```python
from build123d import *

# Parameters (mm, degrees)
SKETCH1_R           = 10
BOSS_EXTRUDE1_DEPTH = 7
SKETCH2_R           = 10
BOSS_EXTRUDE2_DEPTH = 4
SKETCH3_R           = 7
BOSS_EXTRUDE3_DEPTH = 19
SKETCH4_R           = 3
CUT_EXTRUDE1_DEPTH  = 31
CHAMFER1_SIZE       = 0.5
CUT_EXTRUDE2_START  = 10.2
CUT_EXTRUDE2_DEPTH  = 5.8


with BuildPart() as part:
    # Sketch1 → Boss-Extrude1 (new body)
    with BuildSketch(Plane(origin=(0, 0, 0), x_dir=(0, 0, -1), z_dir=(1, 0, 0))):
        Circle(SKETCH1_R)
    extrude(amount=BOSS_EXTRUDE1_DEPTH)

    # Sketch2 → Boss-Extrude2 (add)
    with BuildSketch(Plane(origin=(7, 0, 0), x_dir=(0, 0, -1), z_dir=(1, 0, 0))):
        with Locations((0, 5)):
            Circle(SKETCH2_R)
    extrude(amount=BOSS_EXTRUDE2_DEPTH)

    # Sketch3 → Boss-Extrude3 (add)
    with BuildSketch(Plane(origin=(11, 0, 0), x_dir=(0, 0, -1), z_dir=(1, 0, 0))):
        with Locations((0, 5)):
            Circle(SKETCH3_R)
    extrude(amount=BOSS_EXTRUDE3_DEPTH)

    # Sketch4 → Cut-Extrude1 (cut, through all)
    with BuildSketch(Plane(origin=(30, 0, 0), x_dir=(0, 0, -1), z_dir=(1, 0, 0))):
        with Locations((0, 5)):
            Circle(SKETCH4_R)
    extrude(amount=-CUT_EXTRUDE1_DEPTH, mode=Mode.SUBTRACT)

    # Chamfer1
    chamfer1_edges = [part.edges().sort_by_distance(p)[0] for p in [
        (0, 5, 3),
        (30, 5, 3),
    ]]
    chamfer(chamfer1_edges, length=CHAMFER1_SIZE)

    # Sketch5 → Cut-Extrude2 (cut, through all)
    with BuildSketch(Plane(origin=(0, 0, 0), x_dir=(1, 0, 0), z_dir=(0, 1, 0)).offset(CUT_EXTRUDE2_START)):
        with BuildLine():
            Line((31, 2.5), (18.5, 2.5))
            ThreePointArc((18.5, 2.5), (16, 0), (18.5, -2.5))
            Line((18.5, -2.5), (31, -2.5))
            Line((31, -2.5), (31, 2.5))
        make_face()
    extrude(amount=CUT_EXTRUDE2_DEPTH, mode=Mode.SUBTRACT)


solid = part.part
```
Input: part model. Units: mm. Frame: model coordinates. A direction names the side the tool comes from. Give positions to 0.01 mm unless a question says otherwise; leave off trailing zeros. Loops run counter-clockwise (first coordinate to the right, second up) from the corner with the lowest first, then second, coordinate; pieces in that order, holes last. Notation, with made-up numbers: M -11.75,-38.75 L 10.25,-38.75 A14 cw 10.25,-21.75 Z; hole C 83.25,31.25 d4. An arc over 180 degrees is marked long. Answer as CSV lines item,"result". Start each with the question number.
1. Reachability of faces 4 (the face through (20.37, -1.21, -3.23)), 5 (the face through (7, -6, 0)), 6 (the face through (24, 11, 2.5)), 7 (the face through (7, 10.2, 0.1)) from +Z, -Z, +X, -X, +Y, -Y: full face, straight path, thin tool, end or side. Return the list, or none.
2. Section B-B on x = 20. Return loops of the section in (y, z), plus the area to 3 significant figures.
3. Pull-direction query (Z, two-part tool) for faces 1 (the face through (3.45, -9.76, 2.17)), 2 (the face through (0, 0, 0)), 3 (the face through (15.2, 2.07, 0.65)); classes: released by +Z, released by -Z, zero draft, split by the parting line, or undercut.
4. Section A-A on z = 0. Return loops of the section in (x, y).
5. Section C-C on y = 5. Return loops of the section in (x, z).
6. Pin query (flat end, axial travel): P1, Ø5, axis at x = 21, y = 12, coming from the +Z side; P2, Ø5, axis at x = 17.5, z = 3, coming from the +Y side; P3, Ø12, axis at x = 9.5, y = 12, coming from the -Z side; P4, Ø5, axis at x = 10.5, y = 7.5, coming from the +Z side. Return the tip coordinate at first contact, or that it passes through.
7. Section D-D on y = -3.25. Return loops of the section in (x, z).
8. Line query: L1, parallel to Y at x = 14.75, z = 0; L2, parallel to Y at x = 10.75, z = 0; L3, parallel to X at y = -5.5, z = 5. Output: solid intervals per line, ascending.
Computed values:
1,face 4,"+X"
1,face 5,"+X, -Y"
1,face 6,"+X, +Y"
1,face 7,"-X, +Y"
2,outline,"M 10.2,-2.5 L 10.2,2.5 L 11.54,2.5 A7 ccw long 11.54,-2.5 Z; hole C 5,0 d6"
2,area,"117 mm²"
3,face 1,"split by the parting line"
3,face 2,"zero draft"
3,face 3,"undercut"
4,outline,"M 0,-10 L 7,-10 L 7,-5 L 11,-5 L 11,-2 L 30,-2 L 30,1.5 L 29.5,2 L 0.5,2 L 0,1.5 Z; M 0,8.5 L 0.5,8 L 29.5,8 L 30,8.5 L 30,10.2 L 16,10.2 L 16,12 L 11,12 L 11,15 L 7,15 L 7,10 L 0,10 Z"
5,outline,"M 0,-8.66 L 7,-8.66 L 7,-10 L 11,-10 L 11,-7 L 30,-7 L 30,-3.5 L 29.5,-3 L 0.5,-3 L 0,-3.5 Z; M 0,3.5 L 0.5,3 L 29.5,3 L 30,3.5 L 30,7 L 11,7 L 11,10 L 7,10 L 7,8.66 L 0,8.66 Z"
6,P1,"stops at z = 5.36"
6,P2,"stops at y = 11.94"
6,P3,"stops at z = -9.95"
6,P4,"stops at z = 10"
7,outline,"M 0,-9.46 L 7,-9.46 L 7,-5.65 L 11,-5.65 L 11,5.65 L 7,5.65 L 7,9.46 L 0,9.46 Z"
8,L1,"y = -2 to 2, 8 to 12"
8,L2,"y = -5 to 2, 8 to 15"
8,L3,"x = 0 to 7"
